Answer from the drawing. Dimensions are ordinates in mm from the lowest x, y and z of the part. A direction names the side the tool comes from. Coordinates: 2 decimals unless noted, no trailing zeros. Order: outer loops, then holes, each group sorted by start corner. A loop starts at its lowest first (then second) coordinate and runs counter-clockwise, first axis right, second up. Notation, with made-up numbers: (69, 31.25) - (126, 31.25) arc R29 cw to (126, 60.25) - close; hole circle Ø8 at (63.25, 15.25). An arc over 180 degrees is marked (long way). Use a Markdown table: item, result. Add a question column.
Item 1: The part is cut by section C-C, the plane z = 42.5. Give the vertices of the cut face in (x, y).
Item 2: For the marked faces 1, 2 and 3, determine the directions among +Z, -Z, +X, -X, +Y, -Y from which every point of the face is accessible in a straight line to the end or side of a thin tool.
Item 3: The part is cut by section B-B, the plane y = 3.25. Give the vertices of the cut face in (x, z) (1 decimal).
Item 4: Flat-ended cylindrical pins translate along their axes: P1, Ø1.5, axis at x = 19, y = 5, coming from the +Z side; P2, Ø3, axis at y = 5, z = 11.5, coming from the -X side; P3, Ø1.3, axis at y = 4, z = 29, coming from the +X side (1 decimal). Find the tip coordinate at first contact, or state that the pin passes through.
Item 5: Find the intervals of material crossed by line 1 along Y through (x, z) = (3, 19); line 2 along Z through (x, y) = (37, 3.25); line 3 along X through (y, z) = (5.25, 38) (1 decimal), in increasing order.
Item 6: The part is cut by section A-A, the plane x = 30. Give the vertices of the cut face in (y, z).
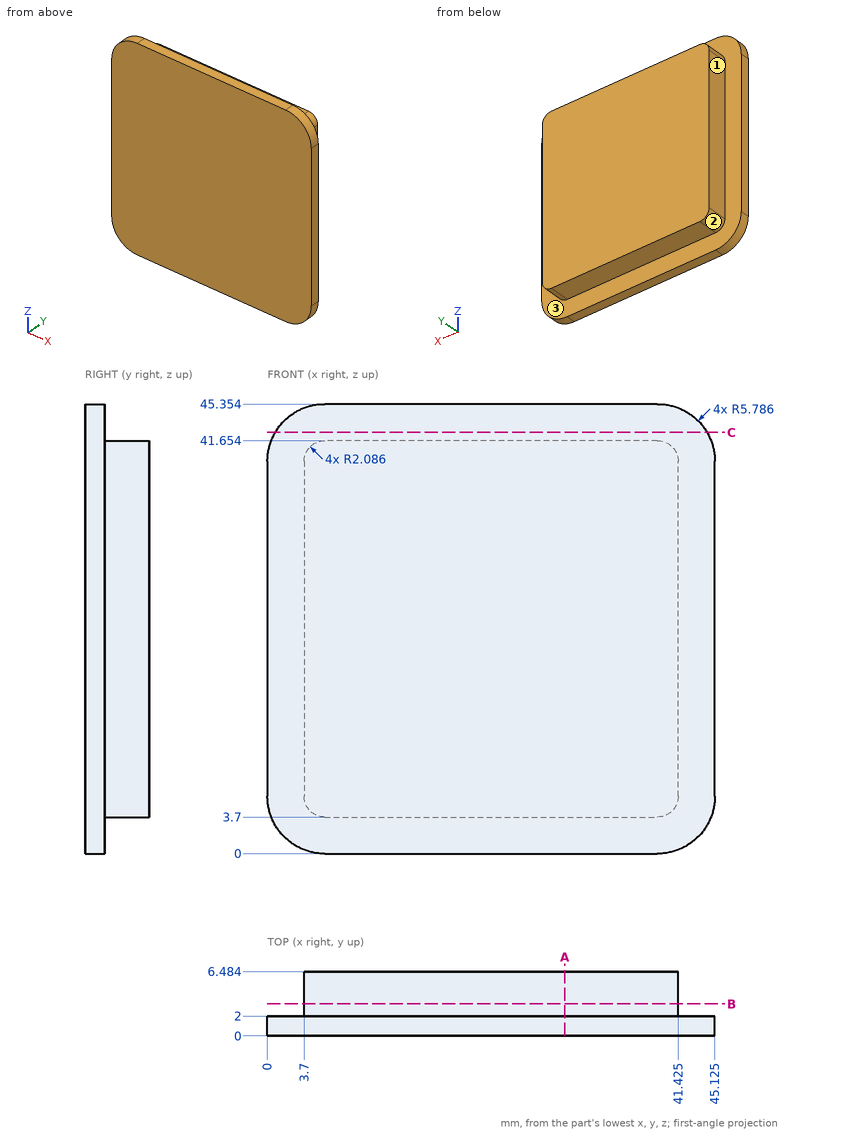
Solution:
| question | item | result |
|---|---|---|
| 1 | outline | (0.8, 0) - (44.33, 0) - (44.33, 2) - (0.8, 2) - close |
| 2 | face 1 | +Z, -Z, -X, +Y |
| 2 | face 2 | -Z, -X, +Y |
| 2 | face 3 | +Y |
| 3 | outline | (3.7, 5.8) arc R2.1 ccw to (5.8, 3.7) - (39.3, 3.7) arc R2.1 ccw to (41.4, 5.8) - (41.4, 39.6) arc R2.1 ccw to (39.3, 41.7) - (5.8, 41.7) arc R2.1 ccw to (3.7, 39.6) - close |
| 4 | P1 | stops at z = 41.65 |
| 4 | P2 | stops at x = 3.7 |
| 4 | P3 | stops at x = 41.4 |
| 5 | line 1 | y = 0 to 2 |
| 5 | line 2 | z = 3.7 to 41.65 |
| 5 | line 3 | x = 3.7 to 41.4 |
| 6 | outline | (0, 0) - (2, 0) - (2, 3.7) - (6.48, 3.7) - (6.48, 41.65) - (2, 41.65) - (2, 45.35) - (0, 45.35) - close |
